```python
from build123d import *

# Parameters (mm, degrees)
F1_DEPTH = 6.35
F2_COUNT = 5
F3_R     = 15
F4_DEPTH = 6.35
F5_R     = 10
F6_DEPTH = 6.351


with BuildPart() as f1:
    # F0 (on Top) → F1 (new body)
    with BuildSketch(Plane.XY):
        with BuildLine():
            Line((0, 38.637033), (0, 0))
            Line((0, 0), (18.929224, 18.929224))
            ThreePointArc((18.929224, 18.929224), (15.818142, 34.885653), (0, 38.637033))
        make_face()
    extrude(amount=F1_DEPTH)



with BuildPart() as f2_1:
    # F2: instance of F1
    add(f1.part.rotate(Axis((0, 0, 3.175), (0, 0, 1)), 1 * 360 / F2_COUNT))


with BuildPart() as f2_2:
    # F2: instance of F1
    add(f1.part.rotate(Axis((0, 0, 3.175), (0, 0, 1)), 2 * 360 / F2_COUNT))


with BuildPart() as f2_3:
    # F2: instance of F1
    add(f1.part.rotate(Axis((0, 0, 3.175), (0, 0, 1)), 3 * 360 / F2_COUNT))


with BuildPart() as f2_4:
    # F2: instance of F1
    add(f1.part.rotate(Axis((0, 0, 3.175), (0, 0, 1)), 4 * 360 / F2_COUNT))


with BuildPart() as f1_1:
    add(f1.part)

    add(f2_1.part)  # F4 merges F2_1

    add(f2_2.part)  # F4 merges F2_2

    add(f2_3.part)  # F4 merges F2_3

    add(f2_4.part)  # F4 merges F2_4
    # F3 (on Top) → F4 (join, through all)
    with BuildSketch(Plane.XY):
        Circle(F3_R)
    extrude(amount=F4_DEPTH)

    # F5 (on face) → F6 (cut, through all)
    with BuildSketch(Plane.XY.offset(6.35)):
        Circle(F5_R)
    extrude(amount=-F6_DEPTH, mode=Mode.SUBTRACT)


solid = f1_1.part
```
The listing builds one solid part. Answer for the finished solid, in the listing's coordinates (mm). A direction names the side the tool comes from. Coordinates: 2 decimals unless noted, no trailing zeros. Write each loop counter-clockwise with the first axis right and the second up, starting at its lowest first coordinate (ties: lowest second). Pieces come first, ordered by that corner, then holes. Notation, with made-up numbers: (63, 79) -> (88, 79) arc R15 cw to (88, 96) -> close; hole circle Ø3 at (70, 41.5). An arc over 180 degrees is marked (long way). Write each question's results on one line, items separated by ' | '. Start each with the question number.
1) Straight lines are drawn through the part: probe 1 along Y at (x, z) = (11.5, 3.5); probe 2 along Y at (x, z) = (-8, 4.25); probe 3 along X at (y, z) = (-15, 5.5). For each, find the intervals that lie inside material, in ascending order.
2) A tool of negligible diameter and unlimited length cuts with its end or side. For faces 1 (the flat face through (-20.546, -3.254, 3.131)), 2 (the flat face through (0, 27, 3)), 3 (the cylindrical face through (7.472, -37.476, 3.131)), 4 (the cylindrical face through (-5.786, -13.839, 3.131)), 5 (the flat face through (10, 2, 6.35)), from which of +Z, -Z, +X, -X, +Y, -Y can it reach the whole face along a straight path? Write none if from no direction.
3) A cutting plane is placed at B-B (x = -16). Determine the outline of the cut face in (y, z), then the cut area to 3 significant figures.
4) For a pull along Y with two mould halves and no side action, classify faces 6 (the flat face through (-15.86, -21.83, 3.13)), 7 (the flat face through (10, 2, 0)), 8 (the flat face through (25.663, 8.339, 3.131)) as +Y half, -Y half, draft (parallel to the pull), parting line (faces both ways), or undercut.
5) Flat-ended cylindrical pins translate along their axes: pin 1 Ø1 at (x, z) = (12, 1) entering from -Y; pin 2 Ø1 at (x, z) = (-25.5, 5.5) entering from +Y; pin 3 Ø3 at (x, z) = (24, 1.5) entering from +Y; pin 4 Ø18 at (x, y) = (0, 0) entering from -Z. Find the tip coordinate at first contact, or state that the pin passes through.
6) A cutting plane is placed at A-A (z = 4.25). Determine the outline of the cut face in (x, y), then the cut area to 3 significant figures.
7) A cutting plane is placed at D-D (x = 27.5). Determine the outline of the cut face in (y, z), then the cut area to 3 significant figures.
8) A cutting plane is placed at C-C (y = 22.5). Determine the outline of the cut face in (x, z).
Values follow:
1) probe 1: -37.71 to -15.83, -9.63 to 9.63, 11.5 to 38.01 | probe 2: -12.69 to -6, 6 to 15.7 | probe 3: -33.32 to -10.9, -2.38 to 10.9
2) face 1: +Z, -Z, -X | face 2: +Z, -Z, +Y | face 3: +Z, -Z, -Y | face 4: +Z, -Z | face 5: +Z, +X, -X, +Y, -Y
3) outline: (-22.02, 0) -> (-2.53, 0) -> (-2.53, 6.35) -> (-22.02, 6.35) -> close; (5.2, 0) -> (26.18, 0) -> (26.18, 6.35) -> (5.2, 6.35) -> close | area: 257 mm²
4) face 6: -Y half | face 7: draft | face 8: undercut
5) pin 1: y = -37.71 | pin 2: y = 26.97 | pin 3: y = 8.29 | pin 4: through
6) outline: (-36.75, 11.94) -> (-14.27, 4.64) arc R15 ccw to (-14.82, -2.35) -> (-26.44, -4.19) arc R15 ccw to (-22.71, -31.26) -> (-8.82, -12.14) arc R15 ccw to (-2.35, -14.82) -> (-4.19, -26.44) arc R15 ccw to (22.71, -31.26) -> (8.82, -12.14) arc R15 ccw to (13.37, -6.81) -> (23.85, -12.15) arc R15 ccw to (36.75, 11.94) -> (14.27, 4.64) arc R15 ccw to (10.61, 10.61) -> (18.93, 18.93) arc R15 ccw to (0, 38.64) -> (0, 15) arc R15 ccw to (-6.81, 13.37) -> (-12.15, 23.85) arc R15 ccw to start; hole circle Ø20 at (0, 0) | area: 2,640 mm²
7) outline: (-11.95, 0) -> (8.94, 0) -> (8.94, 6.35) -> (-11.95, 6.35) -> close | area: 133 mm²
8) outline: (-32.77, 0) -> (-11.46, 0) -> (-11.46, 6.35) -> (-32.77, 6.35) -> close; (0, 0) -> (19.87, 0) -> (19.87, 6.35) -> (0, 6.35) -> close
